Could you check a few things on this drawing? It's one solid part, dimensions in mm from its lowest x, y, z. A direction names the side the tool comes from. Give positions to 0.01 mm unless a question says otherwise; leave off trailing zeros. Loops run counter-clockwise (first coordinate to the right, second up) from the corner with the lowest first, then second, coordinate; pieces in that order, holes last.
Q1. For the marked faces 4 and 5, which set-ups out of +Z, -Z, +X, -X, +Y, -Y let a thin tool reach every point of the face, with its end or its side?
Q2. I'm going to push a flat-ended pin straight in: P1, Ø0.9, axis at x = 15.5, z = 2.5, coming from the -Y side. Where does the tip first touch, or does it pass through?
Q3. Suppose I cut it at A-A (x = 3.5). List the corners of the cut face in (y, z) for me.
Q4. Suppose I cut it at C-C (y = 10.5). List the corners of the cut face in (x, z) for me, and give its area (3 significant figures).
Q5. Suppose I cut it at B-B (z = 2). List the corners of the cut face in (x, y) for me.
Q6. Thinking about a two-plate mould opening in Y: for the marked faces 1, 2 and 3, which applies, pulls with the +Y half, pulls with the -Y half, needs draft (parallel to the pull), parting line crosses it, or undercut?
Q7. Suppose I cut it at D-D (x = 26.5). List the corners of the cut face in (y, z) for me.
Q8. I need wall thicknesses on probe 1 along Y at (x, z) = (26.5, 2.85); probe 2 along X at (y, z) = (1.75, 3.4); probe 3 along Y at (x, z) = (3.5, 3.05). Which ranges of each line are inside material? Lowest first, please.
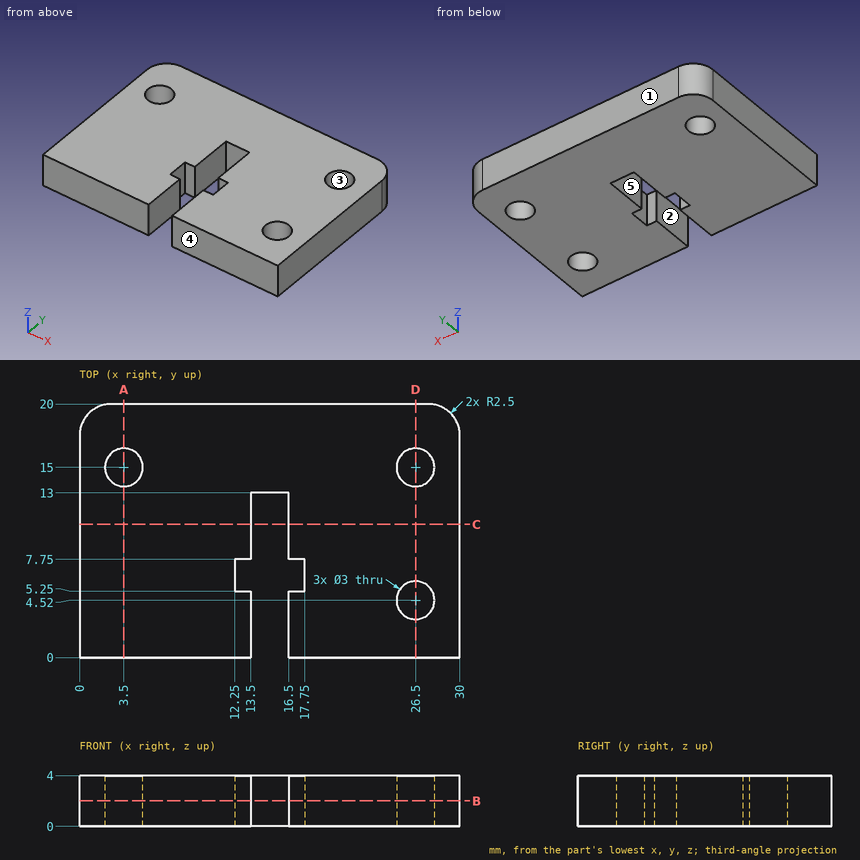
Solutions:
1. face 4: +Z, -Z, +X, -X, -Y
1. face 5: +Z, -Z, -Y
2. P1: stops at y = 13
3. outline: (0, 0) - (13.5, 0) - (13.5, 4) - (0, 4) - close; (16.5, 0) - (20, 0) - (20, 4) - (16.5, 4) - close
4. outline: (0, 0) - (13.5, 0) - (13.5, 4) - (0, 4) - close; (16.5, 0) - (30, 0) - (30, 4) - (16.5, 4) - close
4. area: 108 mm2
5. outline: (0, 0) - (13.5, 0) - (13.5, 5.25) - (12.25, 5.25) - (12.25, 7.75) - (13.5, 7.75) - (13.5, 13) - (16.5, 13) - (16.5, 7.75) - (17.75, 7.75) - (17.75, 5.25) - (16.5, 5.25) - (16.5, 0) - (30, 0) - (30, 17.5) arc R2.5 ccw to (27.5, 20) - (2.5, 20) arc R2.5 ccw to (0, 17.5) - close; hole circle Ø3 at (3.5, 15); hole circle Ø3 at (26.5, 4.52); hole circle Ø3 at (26.5, 15)
6. face 1: pulls with the +Y half
6. face 2: needs draft
6. face 3: undercut
7. outline: (0, 0) - (3.02, 0) - (3.02, 4) - (0, 4) - close; (6.02, 0) - (13.5, 0) - (13.5, 4) - (6.02, 4) - close; (16.5, 0) - (20, 0) - (20, 4) - (16.5, 4) - close
8. probe 1: y = 0 to 3.02, 6.02 to 13.5, 16.5 to 20
8. probe 2: x = 0 to 13.5, 16.5 to 30
8. probe 3: y = 0 to 13.5, 16.5 to 20
